from build123d import *

# Parameters (mm, degrees)
BOSS_EXTRUDE1_DEPTH = 15
CUT_EXTRUDE1_DEPTH  = 5
CUT_EXTRUDE2_DEPTH  = 5
SKETCH4_R           = 0.75
CUT_EXTRUDE3_DEPTH  = 30
CUT_EXTRUDE4_DEPTH  = 5


with BuildPart() as part:
    # Sketch1 → Boss-Extrude1 (new body)
    with BuildSketch(Plane(origin=(0, 0, 0), x_dir=(1, 0, 0), z_dir=(0, 1, 0))):
        Polygon((0, 0), (180, 0), (180, 30), (30, 30), align=None)
    extrude(amount=BOSS_EXTRUDE1_DEPTH)

    # Sketch2 → Cut-Extrude1 (cut)
    with BuildSketch(Plane(origin=(0, 15, 0), x_dir=(1, 0, 0), z_dir=(0, 1, 0))):
        with BuildLine():
            Line((-5, 22.5), (35, 22.5))
            ThreePointArc((35, 22.5), (42.5, 15), (35, 7.5))
            Line((35, 7.5), (-5, 7.5))
            ThreePointArc((-5, 7.5), (-12.5, 15), (-5, 22.5))
        make_face()
        with BuildLine():
            Line((200, 22.5), (160, 22.5))
            ThreePointArc((160, 22.5), (152.5, 15), (160, 7.5))
            Line((160, 7.5), (200, 7.5))
            ThreePointArc((200, 7.5), (207.5, 15), (200, 22.5))
        make_face()
    extrude(amount=-CUT_EXTRUDE1_DEPTH, mode=Mode.SUBTRACT)

    # Sketch3 → Cut-Extrude2 (cut)
    with BuildSketch(Plane.XZ):
        with BuildLine():
            Line((22.5, -22.5), (7.5, -7.5))
            Line((7.5, -7.5), (35, -7.5))
            ThreePointArc((35, -7.5), (42.5, -15), (35, -22.5))
            Line((35, -22.5), (22.5, -22.5))
        make_face()
        with BuildLine():
            Line((180, -7.5), (180, -22.5))
            Line((180, -22.5), (160, -22.5))
            ThreePointArc((160, -22.5), (152.5, -15), (160, -7.5))
            Line((160, -7.5), (180, -7.5))
        make_face()
    extrude(amount=-CUT_EXTRUDE2_DEPTH, mode=Mode.SUBTRACT)

    # Sketch4 → Cut-Extrude3 (cut)
    with BuildSketch(Plane.XY):
        with Locations((90, 7.5)):
            Circle(SKETCH4_R)
        with Locations((45, 7.5)):
            Circle(SKETCH4_R)
        with Locations((135, 7.5)):
            Circle(SKETCH4_R)
    extrude(amount=-CUT_EXTRUDE3_DEPTH, mode=Mode.SUBTRACT)

    # Sketch5 → Cut-Extrude4 (cut)
    with BuildSketch(Plane(origin=(0, 15, 0), x_dir=(1, 0, 0), z_dir=(0, 1, 0))):
        with BuildLine():
            Line((52.5, 25), (142.5, 25))
            ThreePointArc((142.5, 25), (146.035533906, 23.535533906), (147.5, 20))
            Line((147.5, 20), (147.5, 10))
            ThreePointArc((147.5, 10), (146.035533906, 6.464466094), (142.5, 5))
            Line((142.5, 5), (52.5, 5))
            ThreePointArc((52.5, 5), (48.964466094, 6.464466094), (47.5, 10))
            Line((47.5, 10), (47.5, 20))
            ThreePointArc((47.5, 20), (48.964466094, 23.535533906), (52.5, 25))
        make_face()
    extrude(amount=-CUT_EXTRUDE4_DEPTH, mode=Mode.SUBTRACT)


solid = part.part
Build history of the part. All positions in model axes, mm. A direction names the side the tool comes from. Give positions to 0.01 mm unless a question says otherwise; leave off trailing zeros. Order: outer loops, then holes, each group sorted by start corner. A loop starts at its lowest first (then second) coordinate and runs counter-clockwise, first axis right, second up. Notation, with made-up numbers: M 76,-34 L 119,-34 A24 cw 119,-15 Z; hole C 61,-37 d2. An arc over 180 degrees is marked long. Put each result on its own line as item: value.
Item 1: Probe line 1 (Z direction, x = 107, y = 13.25); line 2 (Y direction, x = 90, z = -8); line 3 (Y direction, x = 45, z = -13). List the from-to ranges inside material, lowest first. Write a range as [from, to].
From the geometry:
line 1: z = [-30, -25], [-5, 0]
line 2: y = [0, 6.75], [8.25, 10]
line 3: y = [0, 6.75], [8.25, 15]
Item 2: Flat gauge pins, fed straight in: pin 1 Ø1.4 at (x, y) = (90, 7.5) entering from +Z; pin 2 Ø1.5 at (y, z) = (13, -11) entering from -X; pin 3 Ø4.5 at (x, z) = (160, -14.5) entering from -Y; pin 4 Ø6 at (y, z) = (12.5, -13) entering from -X. Where does each tip first touch, or does it go through?
From the geometry:
pin 1: passes through
pin 2: stops at x = 40.8
pin 3: stops at y = 5
pin 4: stops at x = 11.34
Item 3: Slice it at D-D, the plane x = 128. Write the cut outline in (y, z).
From the geometry:
outline: M 0,-30 L 15,-30 L 15,-25 L 10,-25 L 10,-5 L 15,-5 L 15,0 L 0,0 Z
Item 4: Slice it at C-C, the plane x = 49.5. Write the cut outline in (y, z).
From the geometry:
outline: M 0,-30 L 15,-30 L 15,-24 L 10,-24 L 10,-6 L 15,-6 L 15,0 L 0,0 Z
Item 5: Slice it at B-B, the plane y = 11.5. Write the cut outline in (x, z).
From the geometry:
outline: M 0,0 L 7.5,-7.5 L 35,-7.5 A7.5 cw 35,-22.5 L 22.5,-22.5 L 30,-30 L 180,-30 L 180,-22.5 L 160,-22.5 A7.5 cw 160,-7.5 L 180,-7.5 L 180,0 Z; hole M 47.5,-20 A5 ccw 52.5,-25 L 142.5,-25 A5 ccw 147.5,-20 L 147.5,-10 A5 ccw 142.5,-5 L 52.5,-5 A5 ccw 47.5,-10 Z
Item 6: Two-plate mould, pull along Z, no slides. Class faces 1 (the flat face through (89, 7, 0)), 2 (the flat face through (166, 10, -15)), 3 (the flat face through (106, 7, -30)): +Z half, -Z half, draft (parallel to the pull), parting line (faces both ways), or undercut.
From the geometry:
face 1: +Z half
face 2: undercut
face 3: -Z half
Item 7: 3-axis set-ups, long thin cutter, end or side, ignore diameter. For faces 4 (the flat face through (170, 13, -22.5)), 5 (the cylindrical face through (146.07, 12.54, -6.5)), 6 (the flat face through (170, 2, -22.5)): which of +Z, -Z, +X, -X, +Y, -Y reach the whole face in a straight line?
From the geometry:
face 4: +X, +Y
face 5: +Y
face 6: +X, -Y
Item 8: Slice it at A-A, the plane z = -28. Write the cut outline in (x, y), plus the area to 3 significant figures.
From the geometry:
outline: M 28,0 L 180,0 L 180,15 L 28,15 Z; hole C 45,7.5 d1.5; hole C 90,7.5 d1.5; hole C 135,7.5 d1.5
area: 2,270 mm2
